For this review, take the finished solid that the model builds, in its own axes (mm). Round coordinates to 2 decimals unless told otherwise and drop trailing zeros. Order: outer loops, then holes, each group sorted by start corner. A loop starts at its lowest first (then second) coordinate and runs counter-clockwise, first axis right, second up. Notation, with made-up numbers: (-17, 46.5) -> (-9, 46.5) arc R20 cw to (-9, 50.5) -> close; hole circle Ø3 at (67, 41.25). An arc over 180 degrees is marked (long way). Use a Markdown table: item, result. Add a question column.
1) Consider section A-A (y = -0.25). State the section outline as (x, z) points (1 decimal).
2) Clearance check with a flat-ended pin moving along its axis: P1, Ø5, axis at x = -21.325, z = 31.325, coming from the +Y side. State where the tip first meets the part, or that it passes through.
3) Consider section B-B (z = -42). State the section outline as (x, y) points, plus the area to 3 significant figures.
4) Draft analysis for pull direction Z (two halves, no side actions). For faces 1 (the face through (-19.669, 0.006, -49.775)), 2 (the face through (0, -0.394, -9)), state which applies: pulls with the +Z half, pulls with the -Z half, needs draft (parallel to the pull), parting line crosses it, or undercut.
5) Wall thickness on line 1 along Z through (x, y) = (21.5, 0.2); line 2 along X through (y, z) = (-0.2, -48.5); line 3 along Z through (x, y) = (-19, 0.15): over which ranges is each line inside the solid? List them lowest first. Write a range as [from, to].
Autodesk Inventor part; units mm, degrees
ref_plane "YZ Plane" through (0, 0, 0) normal (1, 0, 0) x (0, 1, 0)
ref_plane "XZ Plane" through (0, 0, 0) normal (0, 1, 0) x (-1, 0, 0)
ref_plane "XY Plane" through (0, 0, 0) normal (0, 0, 1) x (1, 0, 0)
sketch "Sketch1" plane through (0, 0, 0) normal (0, 1, 0) x (-1, 0, 0)
  line L0 (-24.5, 34.5) -> (24.5, 34.5)
  line L1 (24.5, 34.5) -> (24.5, -34.5)
  line L2 (-24.5, -34.5) -> (-24.5, 34.5)
  line L3 (-24.5, 34.5) -> (24.5, -34.5) construction
  line L4 (24.5, 34.5) -> (-24.5, -34.5) construction
  line L5 (22.5, -54.5) -> (-22.5, -54.5)
  line L6 (-22.5, -14.5) -> (22.5, -54.5) construction
  line L7 (22.5, -14.5) -> (-22.5, -54.5) construction
  line L8 (-22.5, -34.5) -> (-22.5, -54.5)
  line L9 (-22.5, -54.5) -> (22.5, -54.5)
  line L10 (22.5, -54.5) -> (22.5, -34.5)
  line L11 (22.5, -34.5) -> (24.5, -34.5)
  line L12 (-24.5, -34.5) -> (-22.5, -34.5)
  line L13 (-22.5, -54.5) -> (-19.325, -54.5)
  line L14 (-19.325, -54.5) -> (-19.325, -51.325)
  line L15 (-19.325, -51.325) -> (-22.5, -51.325)
  line L16 (-22.5, -51.325) -> (-22.5, -54.5)
  point P0 (0, 0)
  point P1 (0, -34.5)
  dimension "d0" = 49
  dimension "d1" = 69
  dimension "d2" = 45
  dimension "d3" = 40
  dimension "d6" = 3.175
  dimension "d7" = 3.175
extrude "Extrusion1" add sketch "Sketch1" along normal mid plane 0.7874
sketch "Sketch2" plane through (0, 0.3937, 0) normal (0, 1, 0) x (1, 0, 0)
  circle A0 centre (-19.325, 51.325) radius 1.5875
  circle A1 centre (19.325, 51.325) radius 1.5875
  circle A2 centre (21.325, -31.325) radius 1.5875
  circle A3 centre (-21.325, -31.325) radius 1.5875
  point P0 (0, 0)
  point P1 (24.5, -34.5)
  point P2 (-22.5, 54.5)
  dimension "d16" = 3.175
  dimension "d17" = 3.175
  dimension "d18" = 3.175
  dimension "d19" = 3.175
extrude "Extrusion2" cut sketch "Sketch2" against normal through all
properties part number "89x49mm-PCB"
Results list:
| question | item | result |
|---|---|---|
| 1 | outline | (-24.5, -34.5) -> (-22.5, -34.5) -> (-22.5, -54.5) -> (22.5, -54.5) -> (22.5, -34.5) -> (24.5, -34.5) -> (24.5, 34.5) -> (-24.5, 34.5) -> close; hole circle Ø3.2 at (-21.3, 31.3); hole circle Ø3.2 at (-19.3, -51.3); hole circle Ø3.2 at (19.3, -51.3); hole circle Ø3.2 at (21.3, 31.3) |
| 2 | P1 | y = 0.39 |
| 3 | outline | (-22.5, -0.39) -> (22.5, -0.39) -> (22.5, 0.39) -> (-22.5, 0.39) -> close |
| 3 | area | 35.4 mm2 |
| 4 | face 1 | undercut |
| 4 | face 2 | needs draft |
| 5 | line 1 | [-54.5, 29.75], [32.9, 34.5] |
| 5 | line 2 | [-22.5, 22.5] |
| 5 | line 3 | [-54.5, -52.88], [-49.77, 34.5] |
